Autodesk Inventor part; units mm, degrees
ref_plane "YZ Plane" through (0, 0, 0) normal (1, 0, 0) x (0, 1, 0)
ref_plane "XZ Plane" through (0, 0, 0) normal (0, 1, 0) x (-1, 0, 0)
ref_plane "XY Plane" through (0, 0, 0) normal (0, 0, 1) x (1, 0, 0)
sketch "Sketch1" plane through (0, 0, 0) normal (0, 1, 0) x (-1, 0, 0)
  line L0 (0, 0) -> (8, 0)
  line L1 (8, 0) -> (8, -67)
  line L2 (8, -67) -> (0, -67)
  line L3 (0, -67) -> (0, 0)
  dimension "d0" = 8
  dimension "d1" = 67
extrude "Extrusion1" add sketch "Sketch1" along normal blind 4.5
sketch "Sketch2" plane through (0, 0, 0) normal (1, 0, 0) x (0, 0, -1)
  line L0 (0, 0) -> (0, 4.5)
  line L1 (0, 4.5) -> (2.25, 4.5)
  line L2 (2.25, 4.5) -> (2.25, 2.25)
  line L3 (2.25, 2.25) -> (0, 2.25)
  line L4 (0, 2.25) -> (0, 4.5)
  circle A0 centre (2.25, 2.25) radius 1.5
  line L5 (67, 0) -> (67, 4.5)
  line L6 (67, 4.5) -> (64.75, 4.5)
  line L7 (64.75, 4.5) -> (64.75, 2.25)
  line L8 (64.75, 2.25) -> (67, 2.25)
  line L9 (67, 2.25) -> (67, 4.5)
  circle A1 centre (64.75, 2.25) radius 1.5
  dimension "d4" = 2.25
  dimension "d5" = 2.25
  dimension "d6" = 3
  dimension "d7" = 2.25
  dimension "d8" = 2.25
  dimension "d9" = 3
extrude "Extrusion2" cut sketch "Sketch2" against normal blind 10 contours A0 L2 L3 | L3 L2 A0 | A1 L7 L8 | L8 L7 A1
properties part number "suport4_pcb_temp"
Geometry: final body of the model. Coordinates: model frame, mm. Round coordinates to 2 decimals unless told otherwise and drop trailing zeros. Write each loop counter-clockwise with the first axis right and the second up, starting at its lowest first coordinate (ties: lowest second). Pieces come first, ordered by that corner, then holes. Notation, with made-up numbers: M 51,-13.5 L 87,-13.5 A28 cw 87,5.5 Z; hole C -10,-21 d1. An arc over 180 degrees is marked long. Answer in a Markdown table with one row per item. Add a question column.
(1) Cut plane C-C, the plane x = -5.5. Return the cut outline in (y, z), then the cut area to 3 significant figures.
(2) Cut plane B-B, the plane z = -2.25. Return the cut outline in (x, y).
(3) Draft query along Y for faces 1 (the face through (-3.94, 2.7, -66.18)), 2 (the face through (-3.944, 0.786, -1.925)), 3 (the face through (-4, 4.5, -33)), 4 (the face through (-4, 2, 0)). Return one class per face: pulls with the +Y half, pulls with the -Y half, needs draft (parallel to the pull), parting line crosses it, or undercut.
(4) Ray query, L1, parallel to Z at x = -3, y = 2.25; L2, parallel to Y at x = -5, z = -64.75; L3, parallel to Y at x = -3.25, z = -63.5. Return the intervals inside material, ascending.
(5) Cut plane A-A, the plane y = 2.25. Return the cut outline in (x, z).
(6) Contact query for a flat-ended pin moving along its axis: pin 1 (2 mm diameter, centred on x = -6.5, z = -19, fed in from -Y). Output: stop coordinate, or through.
Established:
| question | item | result |
|---|---|---|
| 1 | outline | M 0,-67 L 4.5,-67 L 4.5,0 L 0,0 Z; hole C 2.25,-64.75 d3; hole C 2.25,-2.25 d3 |
| 1 | area | 287 mm² |
| 2 | outline | M -8,0 L 0,0 L 0,0.75 L -8,0.75 Z; M -8,3.75 L 0,3.75 L 0,4.5 L -8,4.5 Z |
| 3 | face 1 | undercut |
| 3 | face 2 | undercut |
| 3 | face 3 | pulls with the +Y half |
| 3 | face 4 | needs draft |
| 4 | L1 | -67 to -66.25, -63.25 to -3.75, -0.75 to 0 |
| 4 | L2 | 0 to 0.75, 3.75 to 4.5 |
| 4 | L3 | 0 to 1.42, 3.08 to 4.5 |
| 5 | outline | M -8,-67 L 0,-67 L 0,-66.25 L -8,-66.25 Z; M -8,-63.25 L 0,-63.25 L 0,-3.75 L -8,-3.75 Z; M -8,-0.75 L 0,-0.75 L 0,0 L -8,0 Z |
| 6 | pin 1 | y = 0 |
